Autodesk Inventor part; units mm, degrees
ref_plane "YZ Plane" through (0, 0, 0) normal (1, 0, 0) x (0, 1, 0)
ref_plane "XZ Plane" through (0, 0, 0) normal (0, 1, 0) x (-1, 0, 0)
ref_plane "XY Plane" through (0, 0, 0) normal (0, 0, 1) x (1, 0, 0)
sketch "Skizze1" plane through (0, 0, 0) normal (0, 1, 0) x (-1, 0, 0)
  line L0 (10, 10) -> (-10, 10)
  line L1 (-10, 10) -> (-10, -10)
  line L2 (-10, -10) -> (10, -10)
  line L3 (10, -10) -> (10, 10)
  line L4 (10, 10) -> (-10, -10) construction
  line L5 (-10, 10) -> (10, -10) construction
  point P0 (0, 0)
  dimension "d0" = 20
  dimension "d1" = 20
extrude "Extrusion1" add sketch "Skizze1" along normal blind 34.5
sketch "Skizze2" plane through (0, 0, 0) normal (0, -1, 0) x (1, 0, 0)
  line L0 (-8.9654, -8) -> (-1.6431, -8)
  line L1 (8, 1.6431) -> (8, 9.2)
  line L2 (-10, 10) -> (10, 10)
  line L3 (-10, -10) -> (-10, 10)
  line L4 (8, 10) -> (-10, 10)
  line L5 (-10, 10) -> (-10, -8)
  line L6 (-10, -8) -> (8, -8)
  line L7 (8, -8) -> (8, 10)
  line L8 (10, 10) -> (10, -10)
  line L9 (-10, 10) -> (10, 10)
  line L10 (-10, -10) -> (-10, 10)
  line L11 (10, -10) -> (-10, -10)
  circle A0 centre (-1.6431, 1.6431) radius 9.6431
  point P0 (0, 0)
extrude "Extrusion2" cut sketch "Skizze2" against normal through all contours L0 L6 L7 L1 L2 L8 L11 L3 | A0 L7 L6
sketch "Skizze3" plane through (0, 34.5, 0) normal (0, 1, 0) x (1, 0, 0)
  line L0 (0.9, -9.6) -> (0.9, -12.8936)
  line L1 (0.9, -12.8936) -> (1.9, -12.8936)
  line L2 (1.9, -12.8936) -> (2.4, -11.85)
  line L3 (2.4, -11.85) -> (1.9, -11.85)
  line L4 (1.9, -12.8936) -> (1.9, -9.6)
  line L5 (-2.9, -12.8936) -> (-2.9, -9.6)
  line L6 (-3.9, -9.6) -> (-3.9, -12.8936)
  line L7 (-3.9, -11.85) -> (-4.4, -11.85)
  line L8 (-4.4, -11.85) -> (-3.9, -12.8936)
  line L9 (-3.9, -12.8936) -> (-2.9, -12.8936)
  line L10 (0.9, -12.8936) -> (1.9, -12.8936)
  line L11 (1.9, -12.8936) -> (1.9, -9.6)
  line L12 (1.9, -9.6) -> (0.9, -9.6)
  line L13 (0.9, -9.6) -> (0.9, -12.8936)
  line L14 (-2.9, -12.8936) -> (-3.9, -12.8936)
  line L15 (-3.9, -12.8936) -> (-3.9, -9.6)
  line L16 (-3.9, -9.6) -> (-2.9, -9.6)
  line L17 (-2.9, -9.6) -> (-2.9, -12.8936)
  point P0 (0, 0)
extrude "Extrusion3" add sketch "Skizze3" against normal up to surface (34.5 mm away)
move faces "Verschieben1" translate (0, 2, 0) faces at (-5.181, 34.5, -2)
properties part number "Blank"
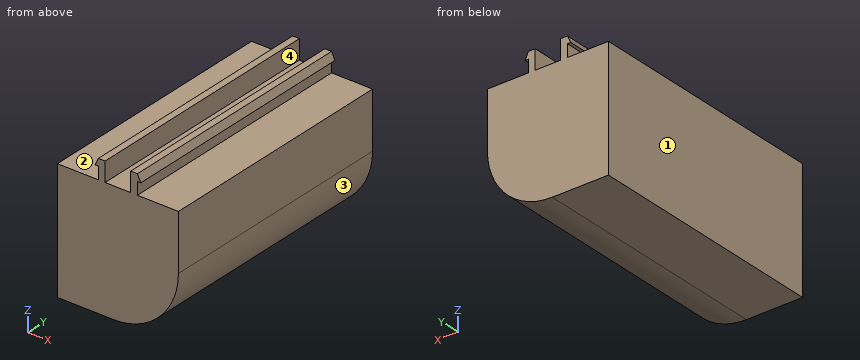
The model under review builds one solid part; all positions refer to its coordinate system, in mm. Face numbers are marked on the shaded views. Round coordinates to 2 decimals unless told otherwise and drop trailing zeros. Write each loop counter-clockwise with the first axis right and the second up, starting at its lowest first coordinate (ties: lowest second). Pieces come first, ordered by that corner, then holes. Notation, with made-up numbers: (52, -30.75) -> (66, -30.75) arc R28 ccw to (66, 0.25) -> close; hole circle Ø3 at (4, 39.5). An arc over 180 degrees is marked (long way). Answer as a JSON object with one key per item and string values.
1. Clearance check with flat-ended pins moving along their axes: pin 1 (0.6 mm diameter, centred on x = 2, y = 18, fed in from -Z); pin 2 (1.5 mm diameter, centred on y = 26.5, z = 0.5, fed in from +X); pin 3 (1.8 mm diameter, centred on x = 6, y = 24.5, fed in from +Z). State where each tip first meets the part, or that it passes through.
Results found:
{"pin 1": "stops at z = -7.4", "pin 2": "stops at x = 7.99", "pin 3": "stops at z = 10"}
2. We need section C-C on x = -2.5. State the section outline as (y, z) points, and give its area (3 significant figures).
Results found:
{"outline": "(0, -8) -> (36.5, -8) -> (36.5, 10) -> (0, 10) -> close", "area": "657 mm^2"}
3. We need section A-A on y = 6. State the section outline as (x, z) points, and give its area (3 significant figures).
Results found:
{"outline": "(-10, -8) -> (-1.64, -8) arc R9.64 ccw to (8, 1.64) -> (8, 10) -> (1.9, 10) -> (1.9, 11.85) -> (2.4, 11.85) -> (1.9, 12.89) -> (0.9, 12.89) -> (0.9, 10) -> (-2.9, 10) -> (-2.9, 12.89) -> (-3.9, 12.89) -> (-4.4, 11.85) -> (-3.9, 11.85) -> (-3.9, 10) -> (-10, 10) -> close", "area": "310 mm^2"}
4. We need section B-B on z = -6.5. State the section outline as (x, y) points, and give its area (3 significant figures).
Results found:
{"outline": "(-10, 0) -> (3.52, 0) -> (3.52, 36.5) -> (-10, 36.5) -> close", "area": "494 mm^2"}
5. The part is to be moulded in two halves that separate along X. For the marked faces 1, 2, 3 and 4, say which applies: pulls with the +X half, pulls with the -X half, needs draft (parallel to the pull), parting line crosses it, or undercut.
Results found:
{"face 1": "pulls with the -X half", "face 2": "needs draft", "face 3": "pulls with the +X half", "face 4": "undercut"}
6. To check wall thickness, follow line 1 along X through (y, z) = (21.5, 10.75); line 2 along Z through (x, y) = (-2, 3); line 3 along Z through (x, y) = (2, 34). State the ranges of each line that lie inside material, in increasing order.
Results found:
{"line 1": "x = -3.9 to -2.9, 0.9 to 1.9", "line 2": "z = -8 to 10", "line 3": "z = -7.29 to 10, 11.85 to 12.68"}
